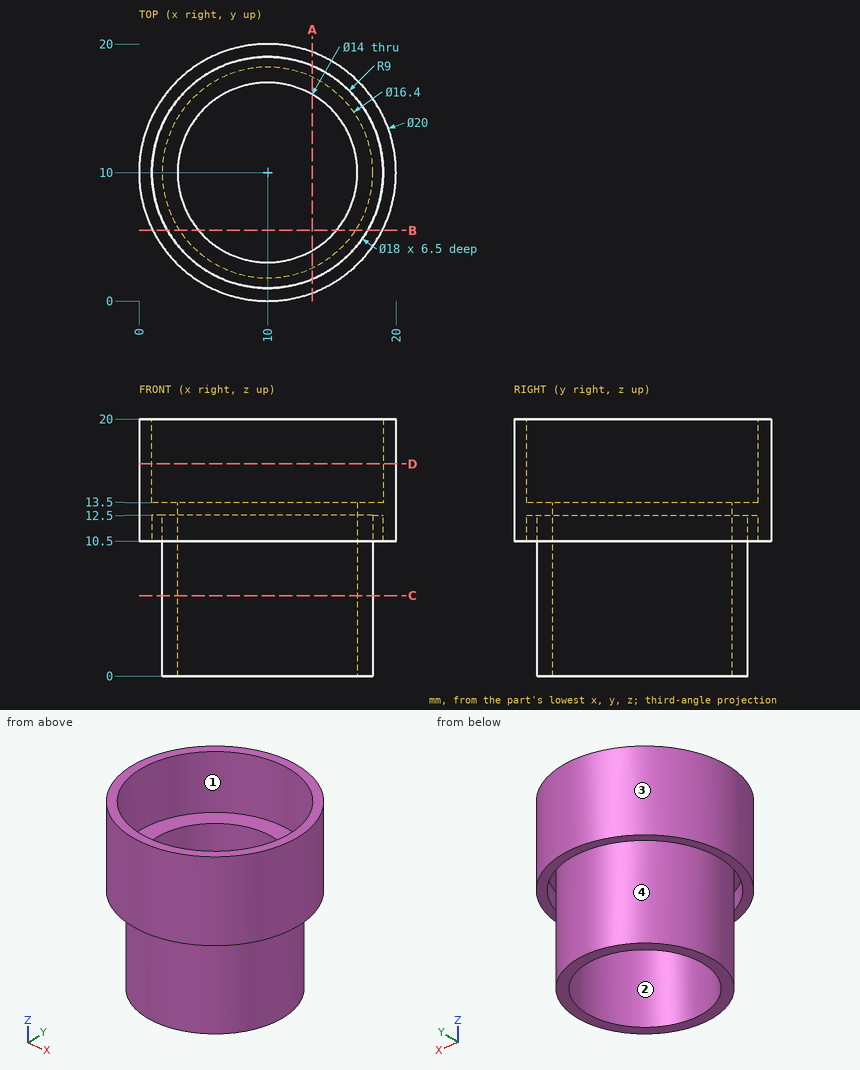
The drawing under review shows one solid part. Ordinate dimensions are in mm from its lowest x, y, z. A direction names the side the tool comes from. Coordinates: 2 decimals unless noted, no trailing zeros. Order: outer loops, then holes, each group sorted by start corner. A loop starts at its lowest first (then second) coordinate and runs counter-clockwise, first axis right, second up. Notation, with made-up numbers: (45, 5) -> (59, 5) arc R23 ccw to (59, 15) -> close; hole circle Ø8 at (23, -34.5). An arc over 180 degrees is marked (long way). One line per item, written item: value.
1) Clearance check with flat-ended pins moving along their axes: P1, Ø5, axis at y = 5.5, z = 18, coming from the +X side; P2, Ø3, axis at x = 12, z = 11, coming from the -Y side; P3, Ø2, axis at y = 14.5, z = 12.5, coming from the -X side. State where each tip first meets the part, or that it passes through.
Output values:
P1: stops at x = 19.8
P2: stops at y = 0.01
P3: stops at x = 0.63
2) We need section C-C, the plane z = 6.25. Give the boundary of the cut face in (x, y).
Output values:
outline: circle Ø16.4 at (10, 10); hole circle Ø14 at (10, 10)
3) Machinability: for the marked faces 1 and 2, which of the approach directions +Z, -Z, +X, -X, +Y, -Y give a long, thin tool a straight path to every point of the face, cutting with its end or side? Answer none if there is none.
Output values:
face 1: +Z
face 2: +Z, -Z
4) To check wall thickness, follow probe 1 along Y at (x, z) = (10, 17.25); probe 2 along X at (y, z) = (9.75, 5). State the ranges of each line that lie inside material, in increasing order. Write a range as [from, to].
Output values:
probe 1: y = [0, 1], [19, 20]
probe 2: x = [1.8, 3], [17, 18.2]
5) We need section B-B, the plane y = 5.5. Give the boundary of the cut face in (x, z), then the cut area to 3 significant figures.
Output values:
outline: (1.07, 10.5) -> (2.21, 10.5) -> (2.21, 12.5) -> (3.15, 12.5) -> (3.15, 0) -> (4.64, 0) -> (4.64, 13.5) -> (2.21, 13.5) -> (2.21, 20) -> (1.07, 20) -> close; (15.36, 0) -> (16.85, 0) -> (16.85, 12.5) -> (17.79, 12.5) -> (17.79, 10.5) -> (18.93, 10.5) -> (18.93, 20) -> (17.79, 20) -> (17.79, 13.5) -> (15.36, 13.5) -> close
area: 63.8 mm2
6) We need section D-D, the plane z = 16.5. Give the boundary of the cut face in (x, y).
Output values:
outline: circle Ø20 at (10, 10); hole circle Ø18 at (10, 10)
7) Draft analysis for pull direction Y (two halves, no side actions). For the marked faces 3 and 4, state which applies: +Y half, -Y half, draft (parallel to the pull), parting line (faces both ways), or undercut.
Output values:
face 3: parting line
face 4: undercut
8) We need section A-A, the plane x = 13.5. Give the boundary of the cut face in (y, z).
Output values:
outline: (0.63, 10.5) -> (1.71, 10.5) -> (1.71, 12.5) -> (2.58, 12.5) -> (2.58, 0) -> (3.94, 0) -> (3.94, 13.5) -> (1.71, 13.5) -> (1.71, 20) -> (0.63, 20) -> close; (16.06, 0) -> (17.42, 0) -> (17.42, 12.5) -> (18.29, 12.5) -> (18.29, 10.5) -> (19.37, 10.5) -> (19.37, 20) -> (18.29, 20) -> (18.29, 13.5) -> (16.06, 13.5) -> close
